from build123d import *

# Parameters (mm, degrees)
ESQUISSE1_W        = 130
ESQUISSE1_H        = 66
ESQUISSE1_R        = 1.5
BOSS_EXTRU_1_DEPTH = 1.5
CONG_1_R           = 1


with BuildPart() as part:
    # Esquisse1 → Boss.-Extru.1 (new body)
    with BuildSketch(Plane(origin=(0, 0, 0), x_dir=(1, 0, 0), z_dir=(0, 1, 0))):
        Rectangle(ESQUISSE1_W, ESQUISSE1_H)
        with Locations(Location((57.5, 24, 0), (0, 0, 270))):
            Circle(ESQUISSE1_R, mode=Mode.SUBTRACT)
        with Locations(Location((-57.5, 24, 0), (0, 0, 90))):
            Circle(ESQUISSE1_R, mode=Mode.SUBTRACT)
        with Locations(Location((-57.5, -24, 0), (0, 0, 270))):
            Circle(ESQUISSE1_R, mode=Mode.SUBTRACT)
        with Locations(Location((57.5, -24, 0), (0, 0, 90))):
            Circle(ESQUISSE1_R, mode=Mode.SUBTRACT)
    extrude(amount=BOSS_EXTRU_1_DEPTH)

    # Congé1
    cong_1_edges = [part.edges().sort_by_distance(p)[0] for p in [
        (-65, 0.75, -33),
        (65, 0.75, -33),
        (65, 0.75, 33),
        (-65, 0.75, 33),
    ]]
    fillet(cong_1_edges, radius=CONG_1_R)


solid = part.part
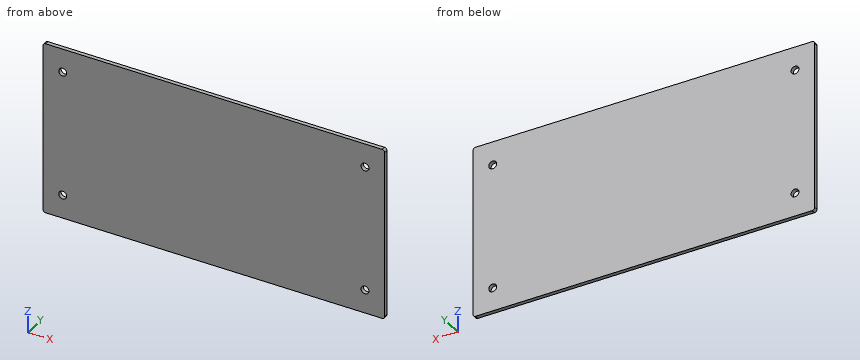
Work out the finished part from the listing and answer in its coordinate system (mm). Coordinates: 2 decimals unless noted, no trailing zeros. Loops run counter-clockwise (first coordinate to the right, second up) from the corner with the lowest first, then second, coordinate; pieces in that order, holes last. Notation, with made-up numbers: M 5,32 L 32,32 A21 ccw 32,62 Z; hole C 38.25,-1 d6. An arc over 180 degrees is marked long. Answer in a Markdown table with one row per item. Add a question column.
1. Consider L1, parallel to X at y = 1, z = -24. Determine where the line is inside the solid, lowest interval first.
2. A flat-ended cylindrical pin translates along its axis: P1, Ø1.8, axis at x = -57.5, z = -24, coming from the -Y side. Find the tip coordinate at first contact, or state that the pin passes through.
3. Find section B-B, the plane z = 24. Write down the section's boundary in (x, y), then the cut area to 3 significant figures.
4. Find section A-A, the plane x = 57.5. Write down the section's boundary in (y, z), then the cut area to 3 significant figures.
Reported:
| question | item | result |
|---|---|---|
| 1 | L1 | x = -65 to -59, -56 to 56, 59 to 65 |
| 2 | P1 | passes through |
| 3 | outline | M -65,0 L -59,0 L -59,1.5 L -65,1.5 Z; M -56,0 L 56,0 L 56,1.5 L -56,1.5 Z; M 59,0 L 65,0 L 65,1.5 L 59,1.5 Z |
| 3 | area | 186 mm^2 |
| 4 | outline | M 0,-33 L 1.5,-33 L 1.5,-25.5 L 0,-25.5 Z; M 0,-22.5 L 1.5,-22.5 L 1.5,22.5 L 0,22.5 Z; M 0,25.5 L 1.5,25.5 L 1.5,33 L 0,33 Z |
| 4 | area | 90.0 mm^2 |
